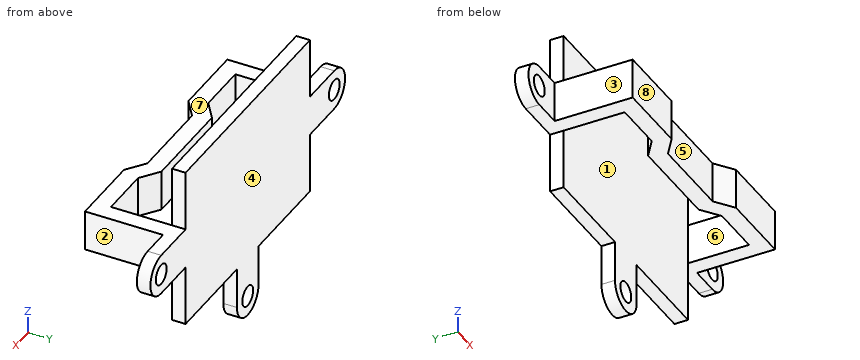
```python
from build123d import *

# Parameters (mm, degrees)
F0_R     = 1.5
F1_DEPTH = 2
F2_W     = 2.5
F2_H     = 6
F3_DEPTH = 9
F5_DEPTH = 3


with BuildPart() as f1:
    # F0 (on Front) → F1 (new body)
    with BuildSketch(Plane.XZ):
        with BuildLine():
            Line((3, -11.95), (17.25, -11.95))
            Line((17.25, -11.95), (17.25, -3))
            Line((17.25, -3), (24, -3))
            ThreePointArc((24, -3), (27, 0), (24, 3))
            Line((24, 3), (17.25, 3))
            Line((17.25, 3), (17.25, 11.95))
            Line((17.25, 11.95), (-17.25, 11.95))
            Line((-17.25, 11.95), (-17.25, 3))
            Line((-17.25, 3), (-24, 3))
            ThreePointArc((-24, 3), (-27, 0), (-24, -3))
            Line((-24, -3), (-17.25, -3))
            Line((-17.25, -3), (-17.25, -11.95))
            Line((-17.25, -11.95), (-3, -11.95))
            Line((-3, -11.95), (-3, -18))
            ThreePointArc((-3, -18), (0, -21), (3, -18))
            Line((3, -18), (3, -11.95))
        make_face()
        with Locations((0, -18)):
            Circle(F0_R, mode=Mode.SUBTRACT)
        with Locations((-24, 0)):
            Circle(F0_R, mode=Mode.SUBTRACT)
        with Locations((24, 0)):
            Circle(F0_R, mode=Mode.SUBTRACT)
    extrude(amount=F1_DEPTH)

    # F2 (on face) → F3 (join)
    with BuildSketch(Plane.XZ.offset(2)):
        with Locations((-18.5, 0)):
            Rectangle(F2_W, F2_H)
        with Locations((18.5, 0)):
            Rectangle(F2_W, F2_H)
    extrude(amount=F3_DEPTH)

    # F4 (on Top) → F5 (join, symmetric)
    with BuildSketch(Plane.XY):
        Polygon((-9.75, -11), (-19.75, -11), (-19.75, -13.5), (-8.93704, -13.5), (-6.18704, -11.5), (0, -11.5), (6.18704, -11.5), (8.93704, -13.5), (19.75, -13.5), (19.75, -11), (9.75, -11), (7, -9), (0, -9), (-7, -9), align=None)
    extrude(amount=F5_DEPTH, both=True)


solid = f1.part
```
The model under review builds one solid part; all positions refer to its coordinate system, in mm. Face numbers are marked on the shaded views. A direction names the side the tool comes from. Round coordinates to 2 decimals unless told otherwise and drop trailing zeros. Loops run counter-clockwise (first coordinate to the right, second up) from the corner with the lowest first, then second, coordinate; pieces in that order, holes last. Notation, with made-up numbers: (75.5, 6.5) - (106.5, 6.5) arc R21 ccw to (106.5, 37.5) - close; hole circle Ø11 at (42, -27.75). An arc over 180 degrees is marked (long way). Use a Markdown table: item, result. Add a question column.
Q1. Add section A-A (z = 0). State the section outline as (x, y) points, plus the area to 3 significant figures.
Q2. Machinability: for the marked faces 1, 2, 3, 4 and 5, which of the approach directions +Z, -Z, +X, -X, +Y, -Y give a long, thin tool a straight path to every point of the face, cutting with its end or side? Answer none if there is none.
Q3. Add section D-D (y = -0.75). State the section outline as (x, z) points, plus the area to 3 significant figures.
Q4. Add section B-B (x = 0). State the section outline as (y, z) points, plus the area to 3 significant figures.
Q5. Insertion check: pin 1 Ø3 at (y, z) = (-11, 4) entering from -X; pin 2 Ø1.6 at (y, z) = (-1.5, 9.5) entering from +X; pin 3 Ø1.6 at (x, y) = (-7, -1) entering from -Z. Each pin has a flat end and moves straight along its axis. Give the tip position at first contact, or say it passes through.
Q6. The part is to be moulded in two halves that separate along Y. For the marked faces 6, 7 and 8, say which applies: pulls with the +Y half, pulls with the -Y half, needs draft (parallel to the pull), parting line crosses it, or undercut.
Q7. For probe 1 along Z at (x, y) = (0, -0.5); probe 2 along Z at (x, y) = (24, -0.7); probe 3 along Y at (x, z) = (9, 10), list the stretches that pass through material, from the lowest coordinate up.
Q8. Add section C-C (y = -5.75). State the section outline as (x, z) points.
Worked answers:
| question | item | result |
|---|---|---|
| 1 | outline | (-27, -2) - (-25.5, -2) - (-25.5, 0) - (-27, 0) - close; (-22.5, -2) - (-19.75, -2) - (-19.75, -13.5) - (-8.94, -13.5) - (-6.19, -11.5) - (6.19, -11.5) - (8.94, -13.5) - (19.75, -13.5) - (19.75, -2) - (22.5, -2) - (22.5, 0) - (-22.5, 0) - close; (25.5, -2) - (27, -2) - (27, 0) - (25.5, 0) - close; hole (-17.25, -11) - (-9.75, -11) - (-7, -9) - (7, -9) - (9.75, -11) - (17.25, -11) - (17.25, -2) - (-17.25, -2) - close |
| 1 | area | 243 mm² |
| 2 | face 1 | +Z, -Z |
| 2 | face 2 | +Z, -Z, +X, -Y |
| 2 | face 3 | +Z, -Z, -X, -Y |
| 2 | face 4 | +Z, -Z, +X, -X, +Y |
| 2 | face 5 | +Z, -Z, -Y |
| 3 | outline | (-24, -3) - (-17.25, -3) - (-17.25, -11.95) - (-3, -11.95) - (-3, -18) arc R3 ccw to (3, -18) - (3, -11.95) - (17.25, -11.95) - (17.25, -3) - (24, -3) arc R3 ccw to (24, 3) - (17.25, 3) - (17.25, 11.95) - (-17.25, 11.95) - (-17.25, 3) - (-24, 3) arc R3 ccw to start; hole circle Ø3 at (-24, 0); hole circle Ø3 at (0, -18); hole circle Ø3 at (24, 0) |
| 3 | area | 963 mm² |
| 4 | outline | (-11.5, -3) - (-9, -3) - (-9, 3) - (-11.5, 3) - close; (-2, -21) - (0, -21) - (0, -19.5) - (-2, -19.5) - close; (-2, -16.5) - (0, -16.5) - (0, 11.95) - (-2, 11.95) - close |
| 4 | area | 74.9 mm² |
| 5 | pin 1 | x = -19.75 |
| 5 | pin 2 | x = 17.25 |
| 5 | pin 3 | z = -11.95 |
| 6 | face 6 | undercut |
| 6 | face 7 | needs draft |
| 6 | face 8 | pulls with the -Y half |
| 7 | probe 1 | -21 to -19.5, -16.5 to 11.95 |
| 7 | probe 2 | -3 to -1.5, 1.5 to 3 |
| 7 | probe 3 | -2 to 0 |
| 8 | outline | (-19.75, -3) - (-17.25, -3) - (-17.25, 3) - (-19.75, 3) - close; (17.25, -3) - (19.75, -3) - (19.75, 3) - (17.25, 3) - close |
